```python
from build123d import *

# Parameters (mm, degrees)
CROQUIS1_R              = 8.5
SALIENTE_EXTRUIR1_DEPTH = 5
CROQUIS2_R              = 3
CORTAR_EXTRUIR1_DEPTH   = 15
CHAFL_N1_SIZE           = 2
CHAFL_N1_SIZE2          = 5.494954839


with BuildPart() as part:
    # Croquis1 → Saliente-Extruir1 (new body)
    with BuildSketch(Plane(origin=(0, 0, 0), x_dir=(1, 0, 0), z_dir=(0, 1, 0))):
        Circle(CROQUIS1_R)
    extrude(amount=SALIENTE_EXTRUIR1_DEPTH)

    # Croquis2 → Cortar-Extruir1 (cut)
    with BuildSketch(Plane(origin=(0, 5, 0), x_dir=(1, 0, 0), z_dir=(0, 1, 0))):
        Circle(CROQUIS2_R)
    extrude(amount=-CORTAR_EXTRUIR1_DEPTH, mode=Mode.SUBTRACT)

    # Chaflán1
    chafl_n1_edges = [part.edges().sort_by_distance(p)[0] for p in [
        (-8.5, 5, 0),
    ]]
    chafl_n1_side = [part.faces().sort_by_distance(p)[0] for p in [
        (-8.5, 2.5, 0),
    ]]
    chamfer(chafl_n1_edges, length=CHAFL_N1_SIZE, length2=CHAFL_N1_SIZE2, reference=chafl_n1_side[0])


solid = part.part
```
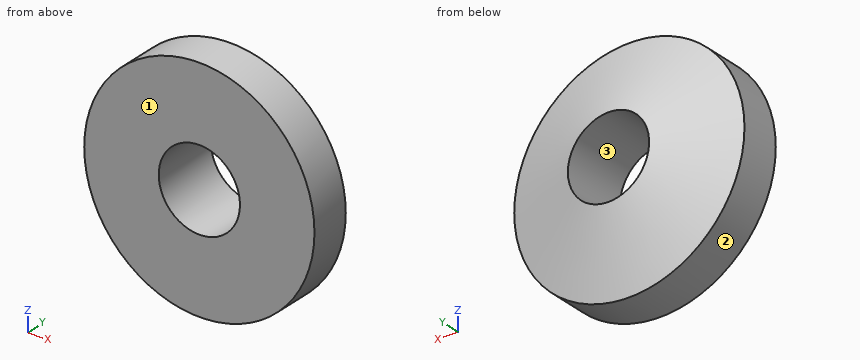
Could you check a few things on this model? Use its own coordinates, in mm. Face numbers are marked on the shaded views. Round coordinates to 2 decimals unless told otherwise and drop trailing zeros. Loops run counter-clockwise (first coordinate to the right, second up) from the corner with the lowest first, then second, coordinate; pieces in that order, holes last. Notation, with made-up numbers: (-31, -19) - (-19, -19) arc R20 cw to (-19, -12) - close; hole circle Ø2 at (-0.5, -27). An arc over 180 degrees is marked (long way). Answer as CSV lines item,"result".
1. We'd pull the mould along Z, two halves only. Please class the marked faces 1, 2 and 3: +Z half, -Z half, draft (parallel to the pull), parting line (faces both ways), or undercut.
Filled in:
face 1,"draft"
face 2,"parting line"
face 3,"undercut"
2. Please list where these lines run through material, in increasing order: line 1 along X through (y, z) = (1.85, 0); line 2 along X through (y, z) = (1.95, -1). Write a range as [from, to].
Filled in:
line 1,"x = [-8.5, -3], [3, 8.5]"
line 2,"x = [-8.44, -2.83], [2.83, 8.44]"
3. For pin 1 Ø3 at (x, y) = (3, 1) entering from -Z; pin 2 Ø1 at (x, y) = (5.5, 3) entering from +Z, each with a flat end and sliding along its axis, tell me the tip position at first contact or that it passes through.
Filled in:
pin 1,"stops at z = -8.37"
pin 2,"stops at z = 6.87"
4. I want a section at C-C on y = 3.3. List the corners of the cut face in (x, z) for me.
Filled in:
outline,"circle Ø15.35 at (0, 0); hole circle Ø6 at (0, 0)"
5. I want a section at B-B on y = 2.15. List the corners of the cut face in (x, z) for me.
Filled in:
outline,"circle Ø17 at (0, 0); hole circle Ø6 at (0, 0)"
